Study the drawing (mm; zero at the part's minimum x, y, z) and answer. A direction names the side the tool comes from. Coordinates: 2 decimals unless noted, no trailing zeros. Order: outer loops, then holes, each group sorted by start corner. A loop starts at its lowest first (then second) coordinate and runs counter-clockwise, first axis right, second up.
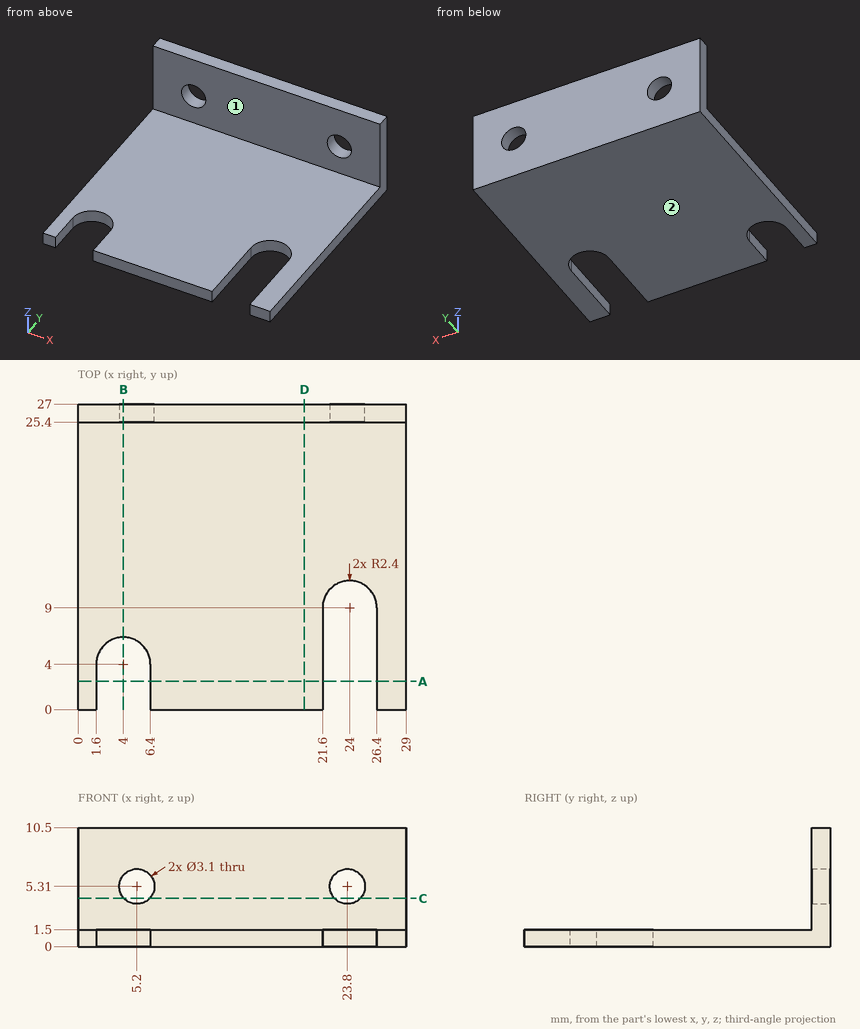
1) Which of the six approach directions +Z, -Z, +X, -X, +Y, -Y give full straight-line access (tool end or side, diameter ignored) to the marked faces 1 and 2?
A:
face 1: +Z, +X, -X, -Y
face 2: -Z, +X, -X, +Y, -Y
2) A cutting plane is placed at B-B, the plane x = 4. Determine the outline of the cut face in (y, z), and give its area (3 significant figures).
A:
outline: (6.4, 0) - (27, 0) - (27, 4.33) - (25.4, 4.33) - (25.4, 1.5) - (6.4, 1.5) - close; (25.4, 6.29) - (27, 6.29) - (27, 10.5) - (25.4, 10.5) - close
area: 42.2 mm2
3) Flat-ended cylindrical pins translate along their axes: pin 1 Ø1 at (x, y) = (19, 17) entering from +Z; pin 2 Ø6 at (x, z) = (21.5, 9) entering from -Y. Find the tip coordinate at first contact, or state that the pin passes through.
A:
pin 1: stops at z = 1.5
pin 2: stops at y = 25.4
4) Straight lines are drawn through the part: line 1 (Z direction, x = 23.8, y = 25.9); line 2 (Z direction, x = 15.25, y = 19.75); line 3 (Y direction, x = 12.75, z = 7). For each, find the intervals that lie inside material, in ascending order.
A:
line 1: z = 0 to 3.76, 6.86 to 10.5
line 2: z = 0 to 1.5
line 3: y = 25.4 to 27
5) A cutting plane is placed at C-C, the plane z = 4.25. Determine the outline of the cut face in (x, y).
A:
outline: (0, 25.4) - (4.07, 25.4) - (4.07, 27) - (0, 27) - close; (6.33, 25.4) - (22.67, 25.4) - (22.67, 27) - (6.33, 27) - close; (24.93, 25.4) - (29, 25.4) - (29, 27) - (24.93, 27) - close
6) A cutting plane is placed at A-A, the plane y = 2.5. Determine the outline of the cut face in (x, z), and give its area (3 significant figures).
A:
outline: (0, 0) - (1.6, 0) - (1.6, 1.5) - (0, 1.5) - close; (6.4, 0) - (21.6, 0) - (21.6, 1.5) - (6.4, 1.5) - close; (26.4, 0) - (29, 0) - (29, 1.5) - (26.4, 1.5) - close
area: 29.1 mm2
7) A cutting plane is placed at D-D, the plane x = 20. Determine the outline of the cut face in (y, z).
A:
outline: (0, 0) - (27, 0) - (27, 10.5) - (25.4, 10.5) - (25.4, 1.5) - (0, 1.5) - close
